Geometry check sheet. Reference: the model listing, model coordinates, mm. Round coordinates to 2 decimals unless told otherwise and drop trailing zeros. Write each loop counter-clockwise with the first axis right and the second up, starting at its lowest first coordinate (ties: lowest second). Pieces come first, ordered by that corner, then holes.
Item 1: Scan lines: probe 1 along Y at (x, z) = (0, 2.3); probe 2 along Y at (x, z) = (-0.5, 2.7); probe 3 along X at (y, z) = (3, 2.45). Record each from-to range of solid material in increasing order.
Item 2: Cross-section at B-B (x = -4). Enter the section's corners in (y, z), then the cut area to 3 significant figures.
Item 3: Depth check by flat-ended pin: P1, Ø1, axis at y = -1.5, z = 2.5, coming from the -X side; P2, Ø1.5, axis at x = 2, y = 3.5, coming from the -Z side. Enter the tip coordinate at first touch or a pass-through.
Item 4: Cross-section at A-A (y = -4.25). Enter the section's corners in (x, z), then the cut area to 3 significant figures.
from build123d import *

# Parameters (mm, degrees)
F1_DEPTH = 3


with BuildPart() as f1:
    # F0 (on Top) → F1 (new body)
    with BuildSketch(Plane.XY):
        Polygon((3.175426, 5.5), (-3.175426, 5.5), (-6.350853, 0), (-3.175426, -5.5), (3.175426, -5.5), (6.350853, 0), align=None)
        with BuildLine():
            ThreePointArc((2.748598, 0.087788), (2.74965, 0.043899), (2.75, 0))
            ThreePointArc((2.75, 0), (2.749649, -0.043966), (2.748594, -0.08792))
            Line((2.748594, -0.08792), (3.146129, -0.201912))
            Line((3.146129, -0.201912), (3.119345, -0.456748))
            Line((3.119345, -0.456748), (2.706787, -0.485596))
            ThreePointArc((2.706787, -0.485596), (2.689892, -0.571822), (2.670251, -0.657464))
            Line((2.670251, -0.657464), (3.035399, -0.851616))
            Line((3.035399, -0.851616), (2.956217, -1.095315))
            Line((2.956217, -1.095315), (2.546676, -1.037758))
            ThreePointArc((2.546676, -1.037758), (2.512223, -1.118586), (2.475205, -1.198273))
            Line((2.475205, -1.198273), (2.792007, -1.464102))
            Line((2.792007, -1.464102), (2.663887, -1.686012))
            Line((2.663887, -1.686012), (2.275263, -1.544564))
            ThreePointArc((2.275263, -1.544564), (2.224758, -1.616463), (2.171981, -1.686712))
            Line((2.171981, -1.686712), (2.426591, -2.012598))
            Line((2.426591, -2.012598), (2.255134, -2.203022))
            Line((2.255134, -2.203022), (1.90441, -1.983865))
            ThreePointArc((1.90441, -1.983865), (1.84006, -2.043693), (1.773831, -2.101434))
            Line((1.773831, -2.101434), (1.955122, -2.473135))
            Line((1.955122, -2.473135), (1.74782, -2.623749))
            Line((1.74782, -2.623749), (1.450326, -2.336462))
            ThreePointArc((1.450326, -2.336462), (1.374943, -2.381603), (1.298156, -2.424313))
            Line((1.298156, -2.424313), (1.398204, -2.825584))
            Line((1.398204, -2.825584), (1.164117, -2.929806))
            Line((1.164117, -2.929806), (0.932855, -2.586945))
            ThreePointArc((0.932855, -2.586945), (0.849734, -2.615426), (0.765745, -2.641237))
            Line((0.765745, -2.641237), (0.780178, -3.054541))
            Line((0.780178, -3.054541), (0.529538, -3.107816))
            Line((0.529538, -3.107816), (0.374614, -2.724365))
            ThreePointArc((0.374614, -2.724365), (0.287387, -2.734942), (0.199868, -2.742727))
            Line((0.199868, -2.742727), (0.128055, -3.15))
            Line((0.128055, -3.15), (-0.128185, -3.15))
            Line((-0.128185, -3.15), (-0.2, -2.742718))
            ThreePointArc((-0.2, -2.742718), (-0.287519, -2.734928), (-0.374745, -2.724347))
            Line((-0.374745, -2.724347), (-0.529666, -3.107789))
            Line((-0.529666, -3.107789), (-0.780306, -3.054514))
            Line((-0.780306, -3.054514), (-0.765873, -2.6412))
            ThreePointArc((-0.765873, -2.6412), (-0.84986, -2.615385), (-0.932979, -2.5869))
            Line((-0.932979, -2.5869), (-1.164237, -2.929753))
            Line((-1.164237, -2.929753), (-1.398323, -2.825531))
            Line((-1.398323, -2.825531), (-1.298273, -2.42425))
            ThreePointArc((-1.298273, -2.42425), (-1.375057, -2.381537), (-1.450438, -2.336392))
            Line((-1.450438, -2.336392), (-1.747925, -2.623672))
            Line((-1.747925, -2.623672), (-1.955227, -2.473058))
            Line((-1.955227, -2.473058), (-1.773932, -2.101348))
            ThreePointArc((-1.773932, -2.101348), (-1.840158, -2.043604), (-1.904506, -1.983773))
            Line((-1.904506, -1.983773), (-2.255221, -2.202924))
            Line((-2.255221, -2.202924), (-2.426679, -2.012501))
            Line((-2.426679, -2.012501), (-2.172063, -1.686607))
            ThreePointArc((-2.172063, -1.686607), (-2.224836, -1.616356), (-2.275338, -1.544454))
            Line((-2.275338, -1.544454), (-2.663953, -1.685898))
            Line((-2.663953, -1.685898), (-2.792073, -1.463988))
            Line((-2.792073, -1.463988), (-2.475263, -1.198154))
            ThreePointArc((-2.475263, -1.198154), (-2.512277, -1.118465), (-2.546726, -1.037635))
            Line((-2.546726, -1.037635), (-2.956257, -1.095191))
            Line((-2.956257, -1.095191), (-3.035439, -0.851492))
            Line((-3.035439, -0.851492), (-2.670283, -0.657335))
            ThreePointArc((-2.670283, -0.657335), (-2.68992, -0.571692), (-2.70681, -0.485466))
            Line((-2.70681, -0.485466), (-3.119359, -0.456618))
            Line((-3.119359, -0.456618), (-3.146143, -0.201782))
            Line((-3.146143, -0.201782), (-2.748598, -0.087788))
            ThreePointArc((-2.748598, -0.087788), (-2.75, 6.6e-05), (-2.748594, 0.08792))
            Line((-2.748594, 0.08792), (-3.146129, 0.201912))
            Line((-3.146129, 0.201912), (-3.119345, 0.456748))
            Line((-3.119345, 0.456748), (-2.706787, 0.485596))
            ThreePointArc((-2.706787, 0.485596), (-2.689892, 0.571822), (-2.670251, 0.657464))
            Line((-2.670251, 0.657464), (-3.035399, 0.851616))
            Line((-3.035399, 0.851616), (-2.956217, 1.095315))
            Line((-2.956217, 1.095315), (-2.546676, 1.037758))
            ThreePointArc((-2.546676, 1.037758), (-2.512223, 1.118586), (-2.475205, 1.198273))
            Line((-2.475205, 1.198273), (-2.792007, 1.464102))
            Line((-2.792007, 1.464102), (-2.663887, 1.686012))
            Line((-2.663887, 1.686012), (-2.275263, 1.544564))
            ThreePointArc((-2.275263, 1.544564), (-2.224758, 1.616463), (-2.171981, 1.686712))
            Line((-2.171981, 1.686712), (-2.426591, 2.012598))
            Line((-2.426591, 2.012598), (-2.255134, 2.203022))
            Line((-2.255134, 2.203022), (-1.90441, 1.983865))
            ThreePointArc((-1.90441, 1.983865), (-1.84006, 2.043693), (-1.773831, 2.101434))
            Line((-1.773831, 2.101434), (-1.955122, 2.473135))
            Line((-1.955122, 2.473135), (-1.74782, 2.623749))
            Line((-1.74782, 2.623749), (-1.450326, 2.336462))
            ThreePointArc((-1.450326, 2.336462), (-1.374943, 2.381603), (-1.298156, 2.424313))
            Line((-1.298156, 2.424313), (-1.398204, 2.825584))
            Line((-1.398204, 2.825584), (-1.164117, 2.929806))
            Line((-1.164117, 2.929806), (-0.932855, 2.586945))
            ThreePointArc((-0.932855, 2.586945), (-0.849734, 2.615426), (-0.765745, 2.641237))
            Line((-0.765745, 2.641237), (-0.780178, 3.054541))
            Line((-0.780178, 3.054541), (-0.529538, 3.107816))
            Line((-0.529538, 3.107816), (-0.374614, 2.724365))
            ThreePointArc((-0.374614, 2.724365), (-0.287387, 2.734942), (-0.199868, 2.742727))
            Line((-0.199868, 2.742727), (-0.128055, 3.15))
            Line((-0.128055, 3.15), (0.128185, 3.15))
            Line((0.128185, 3.15), (0.2, 2.742718))
            ThreePointArc((0.2, 2.742718), (0.287519, 2.734928), (0.374745, 2.724347))
            Line((0.374745, 2.724347), (0.529666, 3.107789))
            Line((0.529666, 3.107789), (0.780306, 3.054514))
            Line((0.780306, 3.054514), (0.765873, 2.6412))
            ThreePointArc((0.765873, 2.6412), (0.84986, 2.615385), (0.932979, 2.5869))
            Line((0.932979, 2.5869), (1.164237, 2.929753))
            Line((1.164237, 2.929753), (1.398323, 2.825531))
            Line((1.398323, 2.825531), (1.298273, 2.42425))
            ThreePointArc((1.298273, 2.42425), (1.375057, 2.381537), (1.450438, 2.336392))
            Line((1.450438, 2.336392), (1.747925, 2.623672))
            Line((1.747925, 2.623672), (1.955227, 2.473058))
            Line((1.955227, 2.473058), (1.773932, 2.101348))
            ThreePointArc((1.773932, 2.101348), (1.840158, 2.043604), (1.904506, 1.983773))
            Line((1.904506, 1.983773), (2.255221, 2.202924))
            Line((2.255221, 2.202924), (2.426679, 2.012501))
            Line((2.426679, 2.012501), (2.172063, 1.686607))
            ThreePointArc((2.172063, 1.686607), (2.224836, 1.616356), (2.275338, 1.544454))
            Line((2.275338, 1.544454), (2.663953, 1.685898))
            Line((2.663953, 1.685898), (2.792073, 1.463988))
            Line((2.792073, 1.463988), (2.475263, 1.198154))
            ThreePointArc((2.475263, 1.198154), (2.512277, 1.118465), (2.546726, 1.037635))
            Line((2.546726, 1.037635), (2.956257, 1.095191))
            Line((2.956257, 1.095191), (3.035439, 0.851492))
            Line((3.035439, 0.851492), (2.670283, 0.657335))
            ThreePointArc((2.670283, 0.657335), (2.68992, 0.571692), (2.70681, 0.485466))
            Line((2.70681, 0.485466), (3.119359, 0.456618))
            Line((3.119359, 0.456618), (3.146143, 0.201782))
            Line((3.146143, 0.201782), (2.748598, 0.087788))
        make_face(mode=Mode.SUBTRACT)
    extrude(amount=F1_DEPTH)


solid = f1.part
Resolved:
1. probe 1: y = -5.5 to -3.15, 3.15 to 5.5
1. probe 2: y = -5.5 to -3.03, 3.03 to 5.5
1. probe 3: x = -4.62 to -0.78, -0.49 to -0.15, 0.15 to 0.49, 0.78 to 4.62
2. outline: (-4.07, 0) - (4.07, 0) - (4.07, 3) - (-4.07, 3) - close
2. area: 24.4 mm2
3. P1: stops at x = -5.77
3. P2: stops at z = 0
4. outline: (-3.9, 0) - (3.9, 0) - (3.9, 3) - (-3.9, 3) - close
4. area: 23.4 mm2
